Geometry check sheet. Reference: the model listing, model coordinates, mm. Round coordinates to 2 decimals unless told otherwise and drop trailing zeros. Order: outer loops, then holes, each group sorted by start corner. A loop starts at its lowest first (then second) coordinate and runs counter-clockwise, first axis right, second up.
(1) Sectioned sample at B-B (y = -43.75). Record the boundary of the cut face in (x, z), plus the area to 3 significant figures.
(2) Material ranges on line 1 along Z through (x, y) = (210, -39.5); line 2 along X through (y, z) = (-38.5, 71.75); line 3 along Y through (x, z) = (106, 63), recorded low to high.
(3) Sectioned sample at C-C (z = 55.25). Record the boundary of the cut face in (x, y).
(4) Sectioned sample at D-D (x = 40.5). Record the boundary of the cut face in (y, z).
(5) Go/stop test with flat-tipped pins: pin 1 (12 mm diameter, centred on x = 66.5, z = 56, fed in from -Y); pin 2 (1.5 mm diameter, centred on x = 170.5, z = 60, fed in from +Y); pin 3 (10 mm diameter, centred on x = 171, z = 56, fed in from +Y); pin 4 (2.5 mm diameter, centred on y = -41, z = 59.5, fed in from -X). Record where each tip stops, or that it passes through.
(6) Release check for a two-part mould opening along Z. For faces 1 (the face through (210, -42, 73.169)), 2 (the face through (220, -42, 63)), 3 (the face through (210.867, -41.721, 59.264)), 4 (the face through (98.6, -39.93, 59.62)) record: +Z half, -Z half, draft (parallel to the pull), parting line (faces both ways), or undercut.
(7) Sectioned sample at A-A (x = 210). Record the boundary of the cut face in (y, z), plus the area to 3 significant figures.
from build123d import *

# Parameters (mm, degrees)
F0_R     = 4
F1_DEPTH = 200
F3_DEPTH = 20
F4_R     = 4
F5_DEPTH = 25


with BuildPart() as f1:
    # F0 (on Right) → F1 (new body)
    with BuildSketch(Plane.YZ):
        with Locations((-41.776799, 63.168682)):
            Circle(F0_R)
    extrude(amount=F1_DEPTH)

    # F2 (on face) → F3 (join)
    with BuildSketch(Plane.YZ.offset(200)):
        with BuildLine():
            Line((-37.776799, 73.168682), (-45.776799, 73.168682))
            Line((-45.776799, 73.168682), (-45.776799, 63.168682))
            ThreePointArc((-45.776799, 63.168682), (-41.776799, 67.168682), (-37.776799, 63.168682))
            Line((-37.776799, 63.168682), (-37.776799, 73.168682))
        make_face()
        with BuildLine():
            ThreePointArc((-37.776799, 63.168682), (-41.776799, 67.168682), (-45.776799, 63.168682))
            ThreePointArc((-45.776799, 63.168682), (-41.776799, 59.168682), (-37.776799, 63.168682))
        make_face()
        with BuildLine():
            ThreePointArc((-37.776799, 63.168682), (-41.776799, 59.168682), (-45.776799, 63.168682))
            Line((-45.776799, 63.168682), (-45.776799, 53.168682))
            Line((-45.776799, 53.168682), (-37.776799, 53.168682))
            Line((-37.776799, 53.168682), (-37.776799, 63.168682))
        make_face()
    extrude(amount=F3_DEPTH)

    # F4 (on face) → F5 (cut)
    with BuildSketch(Plane(origin=(0, -37.776799, 0), x_dir=(-1, 0, 0), z_dir=(0, 1, 0))):
        with Locations((-210, 63.168682)):
            Circle(F4_R)
    extrude(amount=-F5_DEPTH, mode=Mode.SUBTRACT)


solid = f1.part
Answer below:
1. outline: (0, 59.69) - (200, 59.69) - (200, 53.17) - (220, 53.17) - (220, 73.17) - (200, 73.17) - (200, 66.65) - (0, 66.65) - close; hole circle Ø8 at (210, 63.17)
1. area: 1,740 mm2
2. line 1: z = 53.17 to 59.17, 67.17 to 73.17
2. line 2: x = 200 to 220
2. line 3: y = -45.77 to -37.78
3. outline: (200, -45.78) - (220, -45.78) - (220, -37.78) - (200, -37.78) - close
4. outline: circle Ø8 at (-41.78, 63.17)
5. pin 1: stops at y = -45.6
5. pin 2: stops at y = -38.59
5. pin 3: stops at y = -38.42
5. pin 4: stops at x = 0
6. face 1: +Z half
6. face 2: draft
6. face 3: undercut
6. face 4: parting line
7. outline: (-45.78, 53.17) - (-37.78, 53.17) - (-37.78, 59.17) - (-45.78, 59.17) - close; (-45.78, 67.17) - (-37.78, 67.17) - (-37.78, 73.17) - (-45.78, 73.17) - close
7. area: 96.0 mm2
